Check sheet for the modelled part. Datum: model origin and axes. Units: mm. A direction names the side the tool comes from. Give positions to 0.01 mm unless a question says otherwise; leave off trailing zeros. Order: outer loops, then holes, each group sorted by start corner. A loop starts at its lowest first (then second) coordinate and runs counter-clockwise, first axis right, second up.
```python
from build123d import *

# Parameters (mm, degrees)
F0_R     = 1.5
F1_DEPTH = 9
F2_R     = 2.5
F3_DEPTH = 1.5
F4_W     = 1
F4_H     = 1.5
F4_H_2   = 1
F4_W_2   = 1.5
F5_DEPTH = 1


# Not quite as in the source:
# - a fillet or chamfer that OpenCascade refuses, or shapes differently, is made with other operations: its cross-section is extruded or revolved along the edge and cut away or added


with BuildPart() as f1:
    # F0 (on Top) → F1 (new body)
    with BuildSketch(Plane.XY):
        Circle(F0_R)
    extrude(amount=F1_DEPTH)

    # F2 (on face) → F3 (join)
    with BuildSketch(Plane.XY.offset(9)):
        Circle(F2_R)
    extrude(amount=F3_DEPTH)

    # F4 (on face) → F5 (cut)
    with BuildSketch(Plane.XY.offset(10.5)):
        with Locations((0, 1.25)):
            Rectangle(F4_W, F4_H)
        Rectangle(F4_W, F4_H_2)
        with Locations((-1.25, 0)):
            Rectangle(F4_W_2, F4_H_2)
        with Locations((1.25, 0)):
            Rectangle(F4_W_2, F4_H_2)
        with Locations((0, -1.25)):
            Rectangle(F4_W, F4_H)
    extrude(amount=-F5_DEPTH, mode=Mode.SUBTRACT)

    # F6: fillet of radius 1 on 1 edges, made by hand

    # F6_s1 → F6_t2 (revolve, cut)
    with BuildSketch(Plane.XZ):
        with BuildLine():
            ThreePointArc((2.5, 9.5), (2.2071067812, 10.2071067812), (1.5, 10.5))
            Line((1.5, 10.5), (2.5, 10.5))
            Line((2.5, 10.5), (2.5, 9.5))
        make_face()
    revolve(axis=Axis((0, 0, 10.5), (0, 0, 1)), mode=Mode.SUBTRACT)

    # F7: fillet of radius 1 on 1 edges, made by hand

    # F7_s1 → F7_t2 (revolve, cut)
    with BuildSketch(Plane.XZ):
        with BuildLine():
            ThreePointArc((2.5, 9.5), (2.1339745962, 9.1339745962), (1.6339745962, 9))
            Line((1.6339745962, 9), (2.5, 9))
            Line((2.5, 9), (2.5, 9.5))
        make_face()
    revolve(axis=Axis((0, 0, 9), (0, 0, 1)), mode=Mode.SUBTRACT)


solid = f1.part
```
Q1. Go/stop test with flat-tipped pins: P1, Ø1.5, axis at x = -1.5, z = 6.5, coming from the -Y side; P2, Ø1.1, axis at y = 1, z = 10, coming from the +X side; P3, Ø0.8, axis at y = 1, z = 10, coming from the -X side. Record where each tip stops, or that it passes through.
Q2. Sectioned sample at C-C, the plane z = 4.75. Record the cut outline in (x, y).
Q3. Sectioned sample at A-A, the plane x = 0. Record the cut outline in (y, z), plus the area to 3 significant figures.
Q4. Tool access check on faces 1 (the flat face through (0.5, 1, 10)), 2 (the flat face through (-0.9, -0.8, 10.5)). Record the directions out of +Z, -Z, +X, -X, +Y, -Y that give a thin tool (end or side, any length) a straight path to the whole face; none if there is none.
Q5. Material ranges on line 1 (Z direction, x = 0.7, y = 0.1); line 2 (Y direction, x = 0.3, z = 9.75); line 3 (Y direction, x = 1.35, z = 7), recorded low to high.
Q6. Draft check along X on faces 3 (the cylindrical face through (-1.5, 0.07, 4.44)), 4 (the flat face through (0.5, -1, 10)), 5 (the flat face through (0.8, 0.9, 10.5)). Enter one of: pulls with the +X half, pulls with the -X half, needs draft (parallel to the pull), parting line crosses it, or undercut.
Filled in:
1. P1: stops at y = -1.3
1. P2: stops at x = 2.42
1. P3: stops at x = -2.37
2. outline: circle Ø3 at (0, 0)
3. outline: (-2.5, 9.5) arc R1 ccw to (-1.63, 9) - (-1.5, 9) - (-1.5, 0) - (1.5, 0) - (1.5, 9) - (1.63, 9) arc R1 ccw to (2.5, 9.5) arc R1 ccw to (2, 10.37) - (2, 9.5) - (-2, 9.5) - (-2, 10.37) arc R1 ccw to start
3. area: 29.9 mm2
4. face 1: +Z
4. face 2: +Z, +X, -X, +Y, -Y
5. line 1: z = 0 to 9.5
5. line 2: y = -2.45 to -2, 2 to 2.45
5. line 3: y = -0.65 to 0.65
6. face 3: parting line crosses it
6. face 4: undercut
6. face 5: needs draft
